Check sheet for the modelled part. Datum: model origin and axes. Units: mm. A direction names the side the tool comes from. Round coordinates to 2 decimals unless told otherwise and drop trailing zeros. Order: outer loops, then holes, each group sorted by start corner. A loop starts at its lowest first (then second) coordinate and runs counter-clockwise, first axis right, second up.
Q1. Cross-section at C-C on x = 0. Record the cut outline in (y, z), then the cut area to 4 significant figures.
Q2. Cross-section at D-D on x = 22.5. Record the cut outline in (y, z).
Q3. Set-up check for faces 4 (the flat face through (-10, -1, 195)), 5 (the flat face through (10, -1, 195)), 6 (the cylindrical face through (0, -2, 191)), 7 (the cylindrical face through (-0.1, -3.5, 193.7)), 8 (the cylindrical face through (-24.88, -4.46, 194.72)): record each of +Z, -Z, +X, -X, +Y, -Y from which the full face is reachable in a straight line by a thin tool's end or side.
Q4. Scan lines: probe 1 along X at (y, z) = (-6.5, 192.5); probe 2 along X at (y, z) = (-5, 194.5); probe 3 along Y at (x, z) = (-28, 197.25). Record each from-to range of solid material in increasing order.
Q5. Mould release check, pull along Z, two halves, no side actions. Record for faces 1 (the cylindrical face through (-16.421, -4.458, 195.644)), 2 (the flat face through (-33.85, -4.54, 191.97)), 3 (the flat face through (0, -7.5, 193)): +Z half, -Z half, draft (parallel to the pull), parting line (faces both ways), or undercut.
Q6. Cross-section at A-A on z = 189. Record the cut outline in (x, y).
Q7. Depth check by flat-ended pin: P1, Ø1.2, axis at y = -0.5, z = 196.5, coming from the -X side; P2, Ø2.5, axis at x = -25.45, z = 193.33, coming from the -Y side; P3, Ø1, axis at y = -3, z = 196, coming from the -X side; P4, Ø6, axis at x = 27.5, z = 195, coming from the +Y side. Enter the tip coordinate at first touch or a pass-through.
Q8. Cross-section at B-B on y = -6.25. Record the cut outline in (x, z).
from build123d import *

# Parameters (mm, degrees)
BOSS_EXTRUDE3_DEPTH     = 6
BOSS_EXTRUDE3_2_DEPTH   = 6
BOSS_EXTRUDE4_DEPTH     = 7.5
CUT_EXTRUDE1_DEPTH      = 204.131478569
CUT_EXTRUDE1_DEPTH_BACK = 204.131478569
SKETCH4_R               = 1.5


with BuildPart() as part:
    # Sketch2 → Boss-Extrude3 (new body)
    with BuildSketch(Plane(origin=(0, -7.5, 0), x_dir=(1, 0, 0), z_dir=(0, 1, 0))):
        with BuildLine():
            ThreePointArc((-10, -189.73665961), (-21.536552519, -188.775466906), (-32.993153757, -187.113473072))
            Line((-32.993153757, -187.113473072), (-34.729635533, -196.961550602))
            ThreePointArc((-34.729635533, -196.961550602), (-22.408228804, -198.7407137), (-10, -199.749843554))
            Line((-10, -199.749843554), (-10, -189.73665961))
        make_face()
    extrude(amount=BOSS_EXTRUDE3_DEPTH)



with BuildPart() as body_2:
    # Sketch2 → Boss-Extrude3 2 (new body)
    with BuildSketch(Plane(origin=(0, -7.5, 0), x_dir=(1, 0, 0), z_dir=(0, 1, 0))):
        with BuildLine():
            ThreePointArc((32.993153757, -187.113473072), (21.536552519, -188.775466906), (10, -189.73665961))
            Line((10, -189.73665961), (10, -199.749843554))
            ThreePointArc((10, -199.749843554), (22.408228804, -198.7407137), (34.729635533, -196.961550602))
            Line((34.729635533, -196.961550602), (32.993153757, -187.113473072))
        make_face()
    extrude(amount=BOSS_EXTRUDE3_2_DEPTH)


with BuildPart() as part_1:
    add(part.part)

    add(body_2.part)  # Boss-Extrude4 merges body 2
    # Sketch2<3> → Boss-Extrude4 (add)
    with BuildSketch(Plane(origin=(0, -7.5, 0), x_dir=(1, 0, 0), z_dir=(0, 1, 0))):
        with BuildLine():
            ThreePointArc((10, -189.73665961), (0, -190), (-10, -189.73665961))
            Line((-10, -189.73665961), (-10, -199.749843554))
            ThreePointArc((-10, -199.749843554), (0, -200), (10, -199.749843554))
            Line((10, -199.749843554), (10, -189.73665961))
        make_face()
    extrude(amount=BOSS_EXTRUDE4_DEPTH)

    # Sketch3 → hole (revolve, cut)
    with BuildSketch(Plane(origin=(0, 0, 0), x_dir=(1, 0, 0), z_dir=(0, 1, 0))):
        Polygon((3.5, -192.5), (2, -192.5), (2, -180), (0, -180), (0, -195), (3.5, -195), align=None)
    revolve(axis=Axis((0, 0, 0), (0, 0, 1)), mode=Mode.SUBTRACT)

    # Sketch4 → Cut-Extrude1 (cut, two sides: drawn at the far end of the back side and taken through both)
    with BuildSketch(Plane.XZ.offset(7.5).offset(-CUT_EXTRUDE1_DEPTH_BACK)):
        with Locations(Location((25.452607483, 193.331747968, 0), (0, 0, 90))):
            Circle(SKETCH4_R)
        with Locations(Location((16.995369836, 194.257966128, 0), (0, 0, 90))):
            Circle(SKETCH4_R)
        with Locations(Location((-25.452607483, 193.331747968, 0), (0, 0, 90))):
            Circle(SKETCH4_R)
        with Locations(Location((-16.995369836, 194.257966128, 0), (0, 0, 90))):
            Circle(SKETCH4_R)
    extrude(amount=CUT_EXTRUDE1_DEPTH + CUT_EXTRUDE1_DEPTH_BACK, mode=Mode.SUBTRACT)


solid = part_1.part
Results found:
1. outline: (-7.5, 190) - (-2, 190) - (-2, 192.5) - (-3.5, 192.5) - (-3.5, 195) - (0, 195) - (0, 200) - (-7.5, 200) - close
1. area: 61.25 mm2
2. outline: (-7.5, 188.66) - (-1.5, 188.66) - (-1.5, 198.73) - (-7.5, 198.73) - close
3. face 4: +Z, -Z, -X, +Y
3. face 5: +Z, -Z, +X, +Y
3. face 6: -Z, +Y
3. face 7: +Y
3. face 8: +Y, -Y
4. probe 1: x = -33.94 to -26.7, -24.2 to 24.2, 26.7 to 33.94
4. probe 2: x = -34.3 to -26.39, -24.51 to -18.48, -15.52 to 15.52, 18.48 to 24.51, 26.39 to 34.3
4. probe 3: y = -7.5 to -1.5
5. face 1: undercut
5. face 2: -Z half
5. face 3: draft
6. outline: (-33.33, -7.5) - (-19.47, -7.5) - (-19.47, -1.5) - (-33.33, -1.5) - close; (19.47, -7.5) - (33.33, -7.5) - (33.33, -1.5) - (19.47, -1.5) - close
7. P1: stops at x = -10
7. P2: passes through
7. P3: stops at x = -34.65
7. P4: stops at y = -1.5
8. outline: (-34.73, 196.96) - (-32.99, 187.11) arc R190 cw to (32.99, 187.11) - (34.73, 196.96) arc R200 ccw to start; hole circle Ø3 at (-25.45, 193.33); hole circle Ø3 at (-17, 194.26); hole circle Ø3 at (17, 194.26); hole circle Ø3 at (25.45, 193.33)
